The model under review builds one solid part; all positions refer to its coordinate system, in mm. Face numbers are marked on the shaded views. A direction names the side the tool comes from. Give positions to 0.01 mm unless a question says otherwise; leave off trailing zeros. Order: outer loops, then holes, each group sorted by start corner. A loop starts at its lowest first (then second) coordinate and runs counter-clockwise, first axis right, second up. Notation, with made-up numbers: M 45.5,70 L 93.5,70 A10 ccw 93.5,82 Z; hole C -28.75,-33.5 d5. An arc over 180 degrees is marked long. One line per question, with ' | ' between items. Start each with the question number.
1. Wall thickness on L1, parallel to X at y = 0.55, z = 0; L2, parallel to Y at x = 2.5, z = -1.75; L3, parallel to Z at x = -0.75, y = 3: over which ranges is each line inside the solid? List them lowest first.
2. For the marked faces 1 and 2, list the 3-axis set-ups (+Z, -Z, +X, -X, +Y, -Y) from which the entire face can be reached by the end or side of a thin tool; tool diameter is ignored.
3. We need section A-A on x = 0. Write out the cut boundary in (y, z), then the cut area to 3 significant figures.
4. We need section C-C on y = 7. Write out the cut boundary in (x, z), then the cut area to 3 significant figures.
5. Insertion check: P1, Ø0.5, axis at y = 8, z = 10.5, coming from the -X side; P2, Ø1, axis at x = -0.5, y = 7.5, coming from the -Z side; P3, Ø4, axis at y = 3.5, z = -1.5, coming from the -X side; P4, Ø3, axis at x = -2.5, z = 5.5, coming from the +Y side. Each pin has a flat end and moves straight along its axis. Give the tip position at first contact, or say it passes through.
6. We need section B-B on z = 0. Write out the cut boundary in (x, y).
7. We need section D-D on x = -2. Write out the cut boundary in (y, z).
```python
from build123d import *

# Parameters (mm, degrees)
SKETCH_1_R      = 2.5
EXTRUDE_2_DEPTH = 1
EXTRUDE_3_DEPTH = 1
FILLET_1_R      = 1


with BuildPart() as part:
    # Эскиз1 → Бобышка-Вытянуть2 (new body)
    with BuildSketch(Plane(origin=(0, 0, 0), x_dir=(1, 0, 0), z_dir=(0, 1, 0))):
        with BuildLine():
            Line((-2.5, -2.449489743), (-2.5, -10.449489743))
            Line((-2.5, -10.449489743), (2.5, -10.449489743))
            Line((2.5, -10.449489743), (2.5, -2.449489743))
            ThreePointArc((2.5, -2.449489743), (0, 3.5), (-2.5, -2.449489743))
        make_face()
        with Locations(Location((0, 0, 0), (0, 0, 270))):
            Circle(SKETCH_1_R, mode=Mode.SUBTRACT)
    extrude(amount=EXTRUDE_2_DEPTH)

    # Эскиз3 → Бобышка-Вытянуть3 (add)
    with BuildSketch(Plane.XY.offset(10.449489743)):
        with BuildLine():
            Line((2.5, 0), (-2.5, 0))
            Line((-2.5, 0), (-2.5, 8))
            ThreePointArc((-2.5, 8), (0, 10.5), (2.5, 8))
            Line((2.5, 8), (2.5, 0))
        make_face()
        with BuildLine():
            Line((-0.751190727, 7.4), (-0.751190727, 8.6))
            ThreePointArc((-0.751190727, 8.6), (0, 9.351190727), (0.751190727, 8.6))
            Line((0.751190727, 8.6), (0.751190727, 7.4))
            ThreePointArc((0.751190727, 7.4), (0, 6.648809273), (-0.751190727, 7.4))
        make_face(mode=Mode.SUBTRACT)
    extrude(amount=EXTRUDE_3_DEPTH)

    # Скругление1
    fillet_1_edges = [part.edges().sort_by_distance(p)[0] for p in [
        (0, 0, 11.449489743),
        (0, 1, 10.449489743),
    ]]
    fillet(fillet_1_edges, radius=FILLET_1_R)


solid = part.part
```
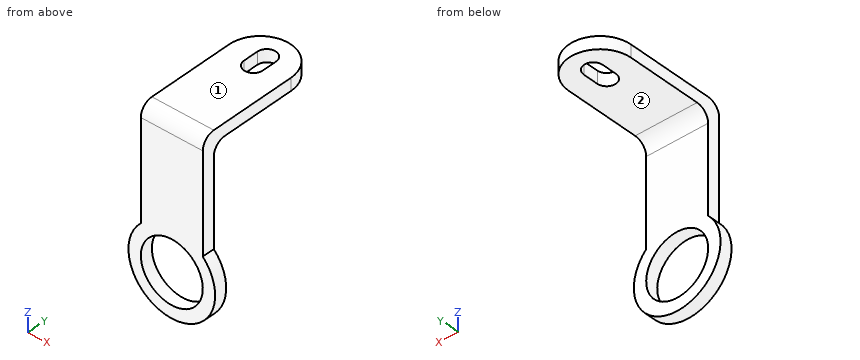
Entries:
1) L1: x = -3.5 to -2.5, 2.5 to 3.5 | L2: y = 0 to 1 | L3: z = 10.45 to 11.45
2) face 1: +Z, +X, -X, +Y, -Y | face 2: -Z, +X, -X, +Y
3) outline: M 0,-3.5 L 1,-3.5 L 1,-2.5 L 0,-2.5 Z; M 0,2.5 L 1,2.5 L 1,9.45 A1 cw 2,10.45 L 6.65,10.45 L 6.65,11.45 L 1,11.45 A1 ccw 0,10.45 Z; M 9.35,10.45 L 10.5,10.45 L 10.5,11.45 L 9.35,11.45 Z | area: 16.7 mm^2
4) outline: M -2.5,10.45 L -0.64,10.45 L -0.64,11.45 L -2.5,11.45 Z; M 0.64,10.45 L 2.5,10.45 L 2.5,11.45 L 0.64,11.45 Z | area: 3.73 mm^2
5) P1: stops at x = -2.5 | P2: stops at z = 10.45 | P3: passes through | P4: stops at y = 1
6) outline: M -3.5,0 L -2.5,0 L -2.5,1 L -3.5,1 Z; M 2.5,0 L 3.5,0 L 3.5,1 L 2.5,1 Z
7) outline: M 0,-2.87 L 1,-2.87 L 1,-1.5 L 0,-1.5 Z; M 0,1.5 L 1,1.5 L 1,9.45 A1 cw 2,10.45 L 9.5,10.45 L 9.5,11.45 L 1,11.45 A1 ccw 0,10.45 Z
